Verification items for the finished model (mm, model axes). Face numbers are marked on the shaded views. A direction names the side the tool comes from. Round coordinates to 2 decimals unless told otherwise and drop trailing zeros. Loops run counter-clockwise (first coordinate to the right, second up) from the corner with the lowest first, then second, coordinate; pieces in that order, holes last. Notation, with made-up numbers: M 56.5,7 L 91.5,7 A31 ccw 91.5,35 Z; hole C 22,89 d4. An arc over 180 degrees is marked long. Answer as CSV lines item,"result".
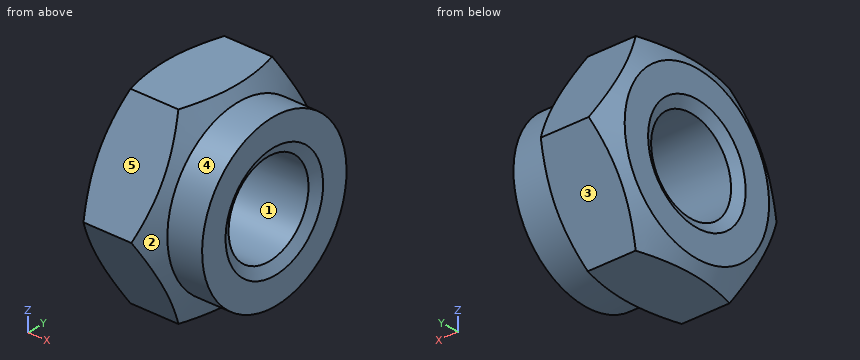
Autodesk Inventor part; units mm, degrees
ref_plane "Work Plane1" through (16.4347, 0, 0) normal (0, 0, 1) x (-1, 0, 0)
ref_plane "YZ Plane" through (0, 0, 0) normal (1, 0, 0) x (0, 1, 0)
ref_plane "XZ Plane" through (0, 0, 0) normal (0, 1, 0) x (-1, 0, 0)
sketch "Sketch1" plane through (0, 0, 0) normal (1, 0, 0) x (0, 1, 0)
  line L0 (2.8868, -5) -> (-2.8868, -5)
  line L1 (-2.8868, -5) -> (-5.7735, 0)
  line L2 (-5.7735, 0) -> (-2.8868, 5)
  line L3 (-2.8868, 5) -> (2.8868, 5)
  line L4 (2.8868, 5) -> (5.7735, 0)
  line L5 (5.7735, 0) -> (2.8868, -5)
  point P0 (0, 0)
  point P1 (0, 0)
  dimension "d0" = 11.547
extrude "Body" add sketch "Sketch1" along normal blind 4.125
sketch "Sketch2" plane through (4.125, 0, 0) normal (1, 0, 0) x (0, 0, -1)
  circle A0 centre (0, 0) radius 4.44
  dimension "d7" = 8.88
extrude "Ring" add sketch "Sketch2" along normal blind 1.875
sketch "Sketch3" plane through (0, 0, 0) normal (0, 0, 1) x (1, 0, 0)
  line L0 (0, 2.8868) -> (0, 5.7735)
  line L1 (0, 5.7735) -> (4.125, 5.7735)
  line L2 (4.125, 2.8868) -> (4.125, 5.7735)
  line L3 (-0.825, 0) -> (4.95, 0)
  line L4 (0, 4.44) -> (0.7699, 5.7735)
  line L5 (3.3551, 5.7735) -> (4.125, 4.44)
  dimension "d3" = 30
  dimension "d4" = 30
  dimension "d5" = 8.88
  dimension "d6" = 8.88
revolve "Chamfer1" cut sketch "Sketch3" angle 360 about axis through (-10, 0, 0) along (1, 0, 0)
sketch "Sketch4" plane through (0, 0, 0) normal (-1, 0, 0) x (0, 0, 1)
  line L0 (0, -8.0829) -> (0, 8.0829)
  line L1 (-7, 0) -> (7, 0)
  point P0 (0, 0)
hole "Thread" at (0, 0, 0) direction (1, 0, 0) diameter 4.917 end through all
chamfer "Chamfer2" distance 0.5413 angle 30 1 edges at (0, 0, -2.4585) measured on face at (0, 3.7305, -0.453)
chamfer "Chamfer3" distance 0.5413 angle 30 1 edges at (6, 0, -2.4585) measured on face at (6, -0.5503, -3.7127)
ref_plane "Work Plane1" through (16.4347, 0, 0) normal (0, 0, 1) x (-1, 0, 0)
equation "\"d0\" = 1.1547 * SW"
equation "\"d1\" = KOH1"
equation "\"d7\" = SD2"
equation "\"d8\" = KOH - KOH1"
equation "\"d3\" = ANG1"
equation "\"d4\" = ANG2"
equation "\"d5\" = SW0"
equation "\"d6\" = SW01"
equation "\"d10\" = -0.5 * GD1 + 0.5 * NND"
equation "\"d46\" = -0.5 * GD1 + 0.5 * NND"
equation "\"d12\" = -0.5 * GD1 + 0.5 * NND"
equation "\"d47\" = -0.5 * GD1 + 0.5 * NND"
equation "\"ANG1\" = 30deg"
equation "\"ANG2\" = 30deg"
equation "\"NND\" = 6"
equation "\"KOH1\" = 4.125"
equation "\"KOH\" = 6"
equation "\"SW0\" = 8.88"
equation "\"SW01\" = SW0"
equation "\"SD2\" = SW0"
equation "\"GUL\" = 0.541266 * PTC"
equation "\"THREADDIA\" = 6"
equation "\"TOA\" = 30deg"
equation "\"PTC\" = 1"
equation "\"KOH1MIN\" = 3.3"
equation "\"E0\" = 1.155 * SW"
equation "\"GAL\" = 0.541266 * PTC"
properties part number "ISO 7042 - M6" material "Steel"
1) Set-up check for the marked faces 4 and 5: record each of +Z, -Z, +X, -X, +Y, -Y from which the full face is reachable in a straight line by a thin tool's end or side.
Here are the results:
face 4,"+X"
face 5,"+Z, +X, -X, -Y"
2) Section check D-D (x = 5.35). Record the cut outline in (y, z), plus the area to 3 significant figures.
Here are the results:
outline,"C 0,0 d8.88; hole C 0,0 d4.92"
area,"42.9 mm^2"
3) Section check B-B (x = 0.6). Record the cut outline in (y, z).
Here are the results:
outline,"M -5.45,-0.56 L -3.21,-4.44 A5.48 ccw -2.24,-5 L 2.24,-5 A5.48 ccw 3.21,-4.44 L 5.45,-0.56 A5.48 ccw 5.45,0.56 L 3.21,4.44 A5.48 ccw 2.24,5 L -2.24,5 A5.48 ccw -3.21,4.44 L -5.45,0.56 A5.48 ccw Z; hole C 0,0 d4.92"
4) Section check C-C (x = 3.05). Record the cut outline in (y, z).
Here are the results:
outline,"M -5.77,0 L -2.89,-5 L 2.89,-5 L 5.77,0 L 2.89,5 L -2.89,5 Z; hole C 0,0 d4.92"
5) Material ranges on probe 1 along Z at (x, y) = (2.55, 0); probe 2 along Z at (x, y) = (4.65, 0); probe 3 along Y at (x, z) = (1.4, -1.75), recorded low to high.
Here are the results:
probe 1,"z = -5 to -2.46, 2.46 to 5"
probe 2,"z = -4.44 to -2.46, 2.46 to 4.44"
probe 3,"y = -4.76 to -1.73, 1.73 to 4.76"
6) Draft check along Z on the marked faces 1, 2 and 3. Enter one of: +Z half, -Z half, draft (parallel to the pull), parting line (faces both ways), or undercut.
Here are the results:
face 1,"undercut"
face 2,"parting line"
face 3,"-Z half"
7) Section check A-A (y = 0). Record the cut outline in (x, z) (1 decimal), plus the area to 3 significant figures.
Here are the results:
outline,"M 0,-4.4 L 0.3,-5 L 3.8,-5 L 4.1,-4.4 L 6,-4.4 L 6,-3 L 5.7,-2.5 L 0.3,-2.5 L 0,-3 Z; M 0,3 L 0.3,2.5 L 5.7,2.5 L 6,3 L 6,4.4 L 4.1,4.4 L 3.8,5 L 0.3,5 L 0,4.4 Z"
area,"27.7 mm^2"
8) Go/stop test with flat-tipped pins: pin 1 (1.5 mm diameter, centred on y = 0, z = -3, fed in from -X); pin 2 (1 mm diameter, centred on x = 1, z = 3, fed in from +Y); pin 3 (1.5 mm diameter, centred on x = 4, y = -4, fed in from +Z). Record where each tip stops, or that it passes through.
Here are the results:
pin 1,"stops at x = 0"
pin 2,"stops at y = 4.33"
pin 3,"stops at z = 4.17"
